The listing builds one solid part. Answer for the finished solid, in the listing's coordinates (mm). Coordinates: 2 decimals unless noted, no trailing zeros. Order: outer loops, then holes, each group sorted by start corner. A loop starts at its lowest first (then second) coordinate and runs counter-clockwise, first axis right, second up. Notation, with made-up numbers: (-27, 66) -> (12, 66) arc R28 cw to (12, 84) -> close; hole circle Ø11 at (14.25, -17.5). An arc over 180 degrees is marked (long way). One line per question, with ' | ' between items.
from build123d import *

# Parameters (mm, degrees)
ESQUISSE10_R                 = 13.380418928
BOSS_EXTRU_1_DEPTH           = 68
BOSS_EXTRU_1_TAPER           = 4
ENL_V_MAT_EXTRU_1_DEPTH      = 68
ENL_V_MAT_EXTRU_1_DEPTH_BACK = 68
ESQUISSE11_R                 = 5
ESQUISSE12_W                 = 2.496707964
ESQUISSE12_H                 = 7.80736829


with BuildPart() as part:
    # Esquisse1 → R_volution1 (revolve)
    with BuildSketch(Plane.XY):
        with BuildLine():
            Line((0, 20), (0, -20))
            ThreePointArc((0, -20), (-20, 0), (0, 20))
        make_face()
    revolve(axis=Axis((0, 20, 0), (0, -1, 0)))

    # Esquisse10 → Boss.-Extru.1 (add)
    with BuildSketch(Plane(origin=(0, 0, 0), x_dir=(1, 0, 0), z_dir=(0, 1, 0))):
        Circle(ESQUISSE10_R)
    extrude(amount=BOSS_EXTRU_1_DEPTH, taper=BOSS_EXTRU_1_TAPER)

    # Esquisse11 → Enl_v. mat.-Extru.1 (cut, two sides: drawn at the far end of the back side and taken through both)
    with BuildSketch(Plane.XY.offset(-ENL_V_MAT_EXTRU_1_DEPTH_BACK)):
        with Locations(Location((0, 56.262547548, 0), (0, 0, 269.999999981))):
            Circle(ESQUISSE11_R)
    extrude(amount=ENL_V_MAT_EXTRU_1_DEPTH + ENL_V_MAT_EXTRU_1_DEPTH_BACK, mode=Mode.SUBTRACT)

    # Balayage1: sweep along a path in Esquisse19
    with BuildLine(Plane(origin=(0, 0, 0), x_dir=(1, 0, 0), z_dir=(0, 1, 0))) as balayage1_path:
        CenterArc((0, 0), 20, 0, 360)
    # Esquisse12 → Balayage1 (sweep)
    with BuildSketch(Plane(origin=(0, 0, 0), x_dir=(0, 0, -1), z_dir=(1, 0, 0))):
        with Locations((-20, 0)):
            Rectangle(ESQUISSE12_W, ESQUISSE12_H)
    sweep(path=balayage1_path.line)


solid = part.part
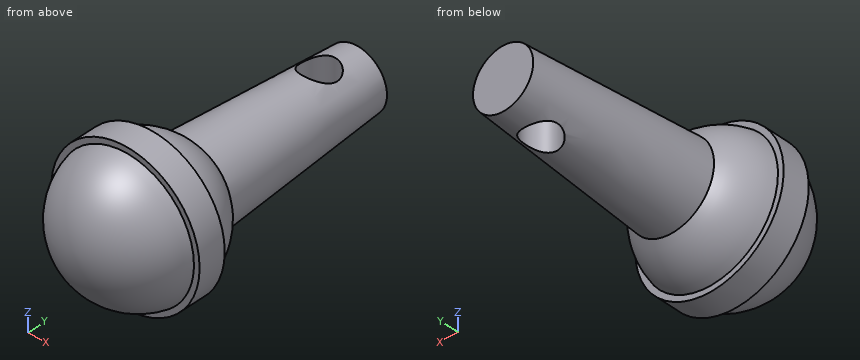
Item 1: Section B-B, the plane y = 10 is taken. Give the vertices of the cut face in (x, z), plus the area to 3 significant figures.
Computed values:
outline: circle Ø34.64 at (0, 0) | area: 942 mm^2
Item 2: Section A-A, the plane y = 63 is taken. Give the vertices of the cut face in (x, z).
Computed values:
outline: circle Ø17.95 at (0, 0)
Item 3: Each of these flat-tipped pins is pushed along its axis until it touches: pin 1 Ø2 at (x, z) = (-14.5, -6.5) entering from +Y; pin 2 Ø6 at (x, y) = (-2, 33) entering from +Z; pin 3 Ø3 at (x, z) = (7.5, -5.5) entering from -Y. Where does it stop, or does it pass through?
Computed values:
pin 1: stops at y = 13.35 | pin 2: stops at z = 11.24 | pin 3: stops at y = -18.42
Item 4: Find the intervals of material crossed by L1, parallel to Y at x = 0, z = 0; L2, parallel to Y at x = 0, z = 4; L3, parallel to X at y = 41, z = 7.5, in increasing order.
Computed values:
L1: y = -20 to 51.26, 61.26 to 68 | L2: y = -19.6 to 51.26, 61.26 to 68 | L3: x = -7.37 to 7.37
